The figure shows three views and two pictorial views of one solid part (mm, origin at its lowest corner). Answer the questions. A direction names the side the tool comes from. Round coordinates to 2 decimals unless told otherwise and drop trailing zeros. Order: outer loops, then holes, each group sorted by start corner. A loop starts at its lowest first (then second) coordinate and runs counter-clockwise, first axis right, second up. Notation, with made-up numbers: M 39.25,-23 L 43.25,-23 A27 ccw 43.25,-6 Z; hole C 2.25,-11.5 d2. An arc over 180 degrees is marked long. Return JSON: item names as keys, results as strings.
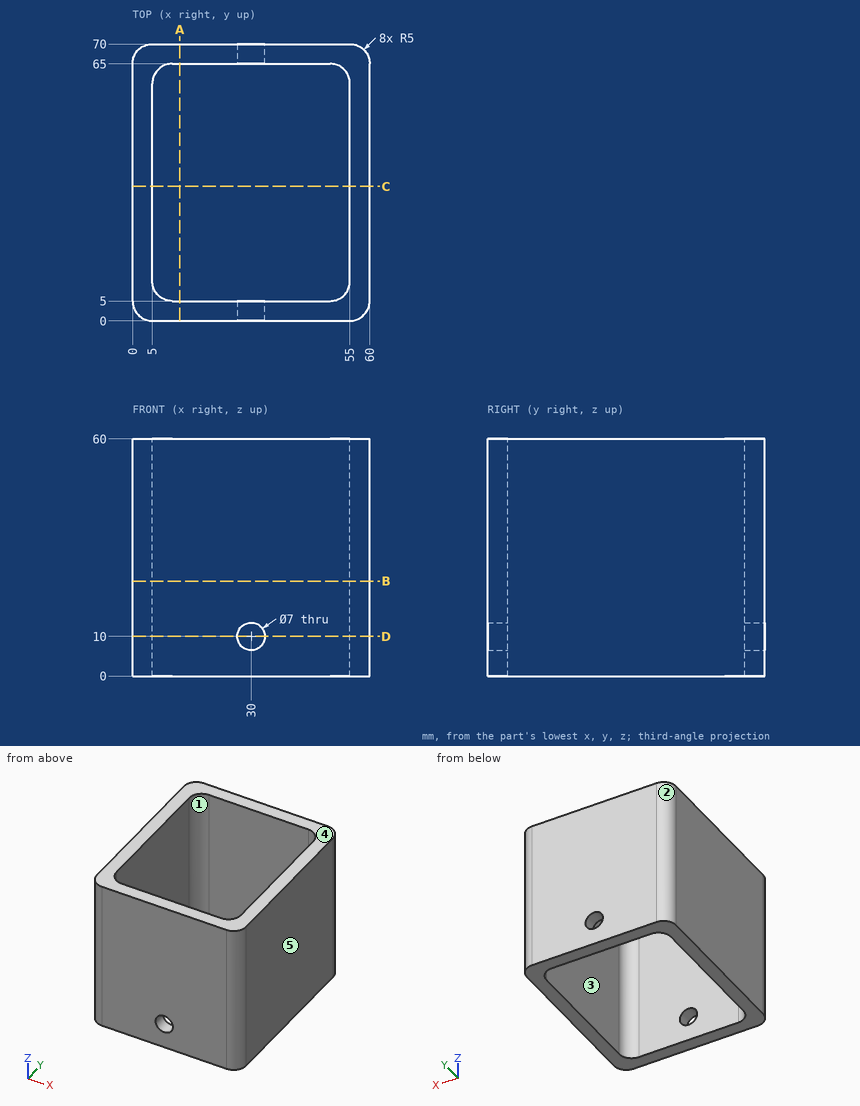
Item 1: Find section A-A (x = 12). Determine the outline of the cut face in (y, z), plus the area to 3 significant figures.
Output:
{"outline": "M 0,0 L 5,0 L 5,60 L 0,60 Z; M 65,0 L 70,0 L 70,60 L 65,60 Z", "area": "600 mm^2"}
Item 2: Find section B-B (z = 24). Determine the outline of the cut face in (x, y).
Output:
{"outline": "M 0,5 A5 ccw 5,0 L 55,0 A5 ccw 60,5 L 60,65 A5 ccw 55,70 L 5,70 A5 ccw 0,65 Z; hole M 5,10 A5 ccw 10,5 L 50,5 A5 ccw 55,10 L 55,60 A5 ccw 50,65 L 10,65 A5 ccw 5,60 Z"}
Item 3: Find section D-D (z = 10). Determine the outline of the cut face in (x, y).
Output:
{"outline": "M 0,5 A5 ccw 5,0 L 26.5,0 L 26.5,5 L 10,5 A5 cw 5,10 L 5,60 A5 cw 10,65 L 26.5,65 L 26.5,70 L 5,70 A5 ccw 0,65 Z; M 33.5,0 L 55,0 A5 ccw 60,5 L 60,65 A5 ccw 55,70 L 33.5,70 L 33.5,65 L 50,65 A5 cw 55,60 L 55,10 A5 cw 50,5 L 33.5,5 Z"}
Item 4: Find section C-C (y = 34). Determine the outline of the cut face in (x, z).
Output:
{"outline": "M 0,0 L 5,0 L 5,60 L 0,60 Z; M 55,0 L 60,0 L 60,60 L 55,60 Z"}
Item 5: Consider line 1 along X through (y, z) = (31, 13); line 2 along Z through (x, y) = (30, 66.9); line 3 along Y through (x, z) = (31, 20.5). Determine where each line is inside the solid, lowest interval first. Write a range as [from, to].
Output:
{"line 1": "x = [0, 5], [55, 60]", "line 2": "z = [0, 6.5], [13.5, 60]", "line 3": "y = [0, 5], [65, 70]"}
Item 6: Which of the six approach directions +Z, -Z, +X, -X, +Y, -Y give full straight-line access (tool end or side, diameter ignored) to the marked faces 1 and 2?
Output:
{"face 1": "+Z, -Z", "face 2": "+Z, -Z, -X, +Y"}
Item 7: The mould has two halves that part along X. Classify the marked faces 3, 4 and 5: pulls with the +X half, pulls with the -X half, needs draft (parallel to the pull), parting line crosses it, or undercut.
Output:
{"face 3": "undercut", "face 4": "needs draft", "face 5": "pulls with the +X half"}
